Work out the finished part from the listing and answer in its coordinate system (mm). Round coordinates to 2 decimals unless told otherwise and drop trailing zeros. Loops run counter-clockwise (first coordinate to the right, second up) from the corner with the lowest first, then second, coordinate; pieces in that order, holes last.
```python
from build123d import *

# Parameters (mm, degrees)
SKETCH9_W           = 12.7
SKETCH9_H           = 25.4
BOSS_EXTRUDE1_DEPTH = 3.175


with BuildPart() as part:
    # Sketch9 → Boss-Extrude1 (new body)
    with BuildSketch(Plane(origin=(0, 0, 0), x_dir=(1, 0, 0), z_dir=(0, 1, 0))):
        with Locations((6.35, 12.7)):
            Rectangle(SKETCH9_W, SKETCH9_H)
    extrude(amount=BOSS_EXTRUDE1_DEPTH)

    # Sketch10 → CSK for M3 SFHCS2 (revolve, cut)
    with BuildSketch(Plane(origin=(6.35, 3.175, -6.35), x_dir=(0, 0, 1), z_dir=(1, 0, 0))):
        Polygon((0, 0), (0, 3.175), (1.7, 3.175), (1.7, 1.66), (3.36, 0), align=None)
    revolve(axis=Axis((6.35, 9.525, -6.35), (0, -1, 0)), mode=Mode.SUBTRACT)


solid = part.part
```
1. Given pin 1 (5 mm diameter, centred on x = 3.5, z = -4, fed in from -Y), flat-ended and moving along its own axis, determine where the tip first touches the part or whether it passes through.
Answer key:
pin 1: stops at y = 0
2. Determine the mould class of faces 1 (the face through (4.917, 0.768, -5.436)), 2 (the face through (6, 2, -25.4)), 3 (the face through (0, 2, -13)) for opening direction Z: +Z half, -Z half, draft (parallel to the pull), parting line (faces both ways), or undercut.
Answer key:
face 1: undercut
face 2: -Z half
face 3: draft
3. Find section C-C (y = 1.9). Write down the section's boundary in (x, z) (3 decimals), then the cut area to 3 significant figures.
Answer key:
outline: (0, -25.4) - (12.7, -25.4) - (12.7, 0) - (0, 0) - close; hole circle Ø4.17 at (6.35, -6.35)
area: 309 mm2
4. Consider probe 1 along X at (y, z) = (0.85, -6.35); probe 2 along Z at (x, y) = (6.35, 0.45); probe 3 along X at (y, z) = (2.55, -5.5). Determine where each line is inside the solid, lowest interval first.
Answer key:
probe 1: x = 0 to 4.65, 8.05 to 12.7
probe 2: z = -25.4 to -8.05, -4.65 to 0
probe 3: x = 0 to 3.75, 8.95 to 12.7
5. Find section B-B (x = 6.35). Write down the section's boundary in (y, z) (3 decimals), then the cut area to 3 significant figures.
Answer key:
outline: (0, -25.4) - (3.175, -25.4) - (3.175, -9.71) - (1.515, -8.05) - (0, -8.05) - close; (0, -4.65) - (1.515, -4.65) - (3.175, -2.99) - (3.175, 0) - (0, 0) - close
area: 67.1 mm2
6. Find section A-A (z = -6.35). Write down the section's boundary in (x, y) (3 decimals).
Answer key:
outline: (0, 0) - (4.65, 0) - (4.65, 1.515) - (2.99, 3.175) - (0, 3.175) - close; (8.05, 0) - (12.7, 0) - (12.7, 3.175) - (9.71, 3.175) - (8.05, 1.515) - close
